The listing builds one solid part. Answer for the finished solid, in the listing's coordinates (mm). Face numbers are marked on the shaded views. A direction names the side the tool comes from. Coordinates: 2 decimals unless noted, no trailing zeros. Order: outer loops, then holes, each group sorted by start corner. A loop starts at its lowest first (then second) coordinate and runs counter-clockwise, first axis right, second up. Notation, with made-up numbers: (61, 87) -> (79, 87) arc R10 cw to (79, 92) -> close; hole circle Ø7 at (2.25, 6). An arc over 180 degrees is marked (long way). Write item = value, one per line.
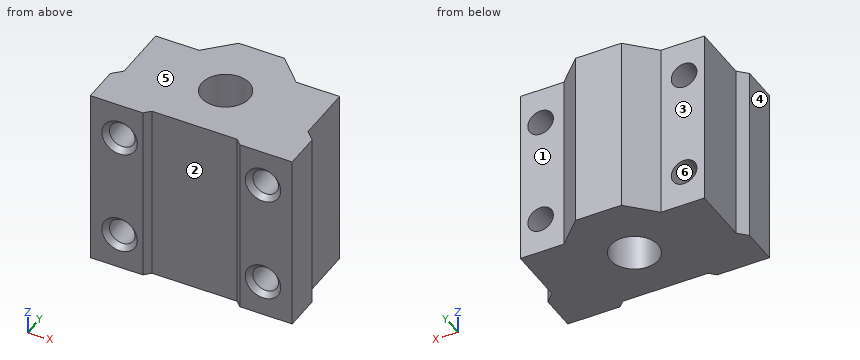
from build123d import *

# Parameters (mm, degrees)
SKETCH1_R                                            = 4
BOSS_EXTRUDE1_DEPTH                                  = 30
CSK_FOR_M4_HEX_SOCKET_COUNTERSUNK_CAP_SC_D           = 4.3
CSK_FOR_M4_HEX_SOCKET_COUNTERSUNK_CAP_SC_CSINK_D     = 5.96
CSK_FOR_M4_HEX_SOCKET_COUNTERSUNK_CAP_SC_CSINK_ANGLE = 90


with BuildPart() as part:
    # Sketch1 → Boss-Extrude1 (new body)
    with BuildSketch(Plane.XY):
        Polygon((0, 0), (0, 6.15), (1.5, 7.65), (1.5, 17.4), (8.8, 17.4), (13.1, 21.7), (20.8, 21.7), (25.1, 17.4), (32.4, 17.4), (32.4, 7.65), (33.9, 6.15), (33.9, 0), (25.1, 0), (24.1, 1), (9.8, 1), (8.8, 0), align=None)
        with Locations((16.95, 10.6)):
            Circle(SKETCH1_R, mode=Mode.SUBTRACT)
    extrude(amount=BOSS_EXTRUDE1_DEPTH)

    # CSK for M4 Hex Socket Countersunk Cap Screw1 (through all)
    with Locations(Plane(origin=(0, 0, 0), x_dir=(-1, 0, 0), z_dir=(0, -1, 0))):
        with Locations((-4.9, -6.05), (-4.9, -23.95), (-29, -6.05), (-29, -23.95)):
            CounterSinkHole(CSK_FOR_M4_HEX_SOCKET_COUNTERSUNK_CAP_SC_D / 2, CSK_FOR_M4_HEX_SOCKET_COUNTERSUNK_CAP_SC_CSINK_D / 2, counter_sink_angle=CSK_FOR_M4_HEX_SOCKET_COUNTERSUNK_CAP_SC_CSINK_ANGLE)


solid = part.part
Q1. A tool of negligible diameter and unlimited length cuts with its end or side. For the marked faces 1, 2 and 3, from which of +Z, -Z, +X, -X, +Y, -Y can it reach the whole face along a straight path? Write none if from no direction.
The answers:
face_1 = +Z, -Z, +X, +Y
face_2 = +Z, -Z, -Y
face_3 = +Z, -Z, -X, +Y
Q2. Section D-D, the plane x = 18 is taken. Give the vertices of the cut face in (y, z), plus the area to 3 significant figures.
The answers:
outline = (1, 0) -> (6.74, 0) -> (6.74, 30) -> (1, 30) -> close; (14.46, 0) -> (21.7, 0) -> (21.7, 30) -> (14.46, 30) -> close
area = 389 mm2
Q3. Section A-A, the plane y = 10.6 is taken. Give the vertices of the cut face in (x, z).
The answers:
outline = (1.5, 0) -> (12.95, 0) -> (12.95, 30) -> (1.5, 30) -> close; (20.95, 0) -> (32.4, 0) -> (32.4, 30) -> (20.95, 30) -> close; hole circle Ø4.3 at (4.9, 6.05); hole circle Ø4.3 at (4.9, 23.95); hole circle Ø4.3 at (29, 6.05); hole circle Ø4.3 at (29, 23.95)
Q4. Each of these flat-tipped pins is pushed along its axis until it touches: pin 1 Ø3 at (y, z) = (13.5, 13.5) entering from -X; pin 2 Ø5.5 at (x, z) = (4.9, 6.05) entering from +Y; pin 3 Ø10 at (y, z) = (12.5, 7) entering from -X. Where does it stop, or does it pass through?
The answers:
pin_1 = 1.5
pin_2 = 17.4
pin_3 = 1.35
Q5. Section C-C, the plane z = 23.95 is taken. Give the number of separate pieces and of enclosed holes in the cut face, plus the area to 3 significant figures.
The answers:
separate_pieces = 3
enclosed_holes = 1
area = 393 mm2
Q6. The mould has two halves that part along Z. Classify the marked faces 4, 5 and 6: released by +Z, released by -Z, zero draft, split by the parting line, or undercut.
The answers:
face_4 = zero draft
face_5 = released by +Z
face_6 = undercut
Q7. Section B-B, the plane x = 29 is taken. Give the vertices of the cut face in (y, z).
The answers:
outline = (0, 0) -> (17.4, 0) -> (17.4, 3.9) -> (0.83, 3.9) -> (0, 3.07) -> close; (0, 9.03) -> (0.83, 8.2) -> (17.4, 8.2) -> (17.4, 21.8) -> (0.83, 21.8) -> (0, 20.97) -> close; (0, 26.93) -> (0.83, 26.1) -> (17.4, 26.1) -> (17.4, 30) -> (0, 30) -> close
Q8. Find the intervals of material crossed by line 1 along Z through (x, y) = (4.9, 9.5); line 2 along Z through (x, y) = (5.5, 13.5); line 3 along Y through (x, z) = (17, 6.75), in increasing order.
The answers:
line_1 = 0 to 3.9, 8.2 to 21.8, 26.1 to 30
line_2 = 0 to 3.99, 8.11 to 21.89, 26.01 to 30
line_3 = 1 to 6.6, 14.6 to 21.7
